Geometry: final body of the model. Coordinates: model frame, mm. Face numbers are marked on the shaded views. A direction names the side the tool comes from. Round coordinates to 2 decimals unless told otherwise and drop trailing zeros. Loops run counter-clockwise (first coordinate to the right, second up) from the corner with the lowest first, then second, coordinate; pieces in that order, holes last. Notation, with made-up numbers: (-10.5, 12.5) - (26.5, 12.5) arc R17 ccw to (26.5, 37.5) - close; hole circle Ø11 at (-14, 66). An arc over 180 degrees is marked (long way). Answer in a Markdown table with one row per item. Add a question column.
from build123d import *

# Parameters (mm, degrees)
F2_SIZE  = 1.5
F3_R     = 7
F4_DEPTH = 75.001


# Not quite as in the source:
# - a feature names something its author has since deleted; it is built from what else it names


with BuildPart() as f1:
    # F0 (on Top) → F1 (revolve)
    with BuildSketch(Plane.XY):
        with BuildLine():
            Line((-18.3783795104, 0), (31.6216204896, 0))
            Line((31.6216204896, 0), (31.6216204896, 11.5))
            Line((31.6216204896, 11.5), (53.6216204896, 11.5))
            Line((53.6216204896, 11.5), (53.6216204896, 15.2837846328))
            Line((53.6216204896, 15.2837846328), (53.6216204896, 25.2837846328))
            Line((53.6216204896, 25.2837846328), (51.6216204896, 25.2837846328))
            Line((51.6216204896, 25.2837846328), (51.6216204896, 15.2837846328))
            Line((51.6216204896, 15.2837846328), (39.6216204896, 15.2837846328))
            Line((39.6216204896, 15.2837846328), (-41.3783795104, 15.2837846328))
            Line((-41.3783795104, 15.2837846328), (-41.3783795104, 17.2837846328))
            Line((-41.3783795104, 17.2837846328), (-43.3783795104, 17.2837846328))
            Line((-43.3783795104, 17.2837846328), (-43.3783795104, 15.2837846328))
            Line((-43.3783795104, 15.2837846328), (-43.3783795104, 11.5))
            Line((-43.3783795104, 11.5), (-28.3783795104, 11.5))
            ThreePointArc((-28.3783795104, 11.5), (-21.3073116985, 8.5710678119), (-18.3783795104, 1.5))
            Line((-18.3783795104, 1.5), (-18.3783795104, 0))
        make_face()
    revolve(axis=Axis((6.6216204896, 0, 0), (-1, 0, 0)))

    # F2
    f2_edges = [f1.edges().sort_by_distance(p)[0] for p in [
        (-41.37838, -17.283785, 0),
    ]]
    chamfer(f2_edges, length=F2_SIZE)

    # F3 (on face) → F4 (cut, through all)
    with BuildSketch(Plane.YZ.offset(31.6216204896)):
        Circle(F3_R)
    extrude(amount=-F4_DEPTH, mode=Mode.SUBTRACT)


solid = f1.part
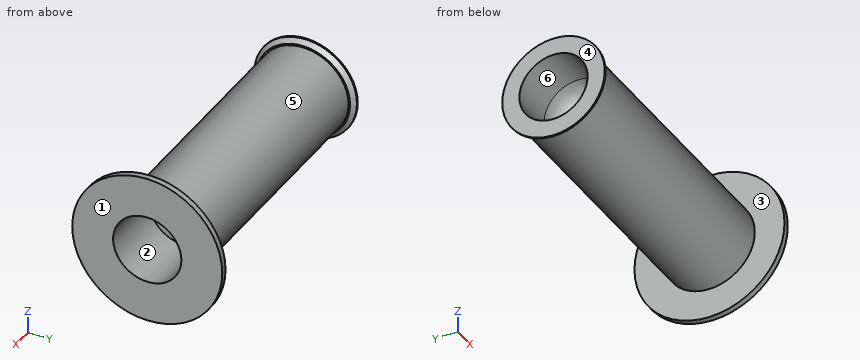
1) Pull-direction query (Z, two-part tool) for the marked faces 4, 5 and 6; classes: pulls with the +Z half, pulls with the -Z half, needs draft (parallel to the pull), parting line crosses it, or undercut.
2) Material intervals for line 1 along Z through (x, y) = (-34, 0); line 2 along Z through (x, y) = (13, 0), sorted ascending. Write a range as from..to.
3) Contact query for flat-ended pins moving along their axis: pin 1 Ø4 at (x, z) = (16.5, -16) entering from +Y; pin 2 Ø10 at (x, y) = (-21.5, 18) entering from -Z; pin 3 Ø5 at (x, y) = (33.5, -1) entering from -Z. Output: stop coordinate, or through.
4) Section B-B, the plane y = 22. Return the cut outline in (x, z), and give its area (3 significant figures).
5) Reachability of the marked faces 1, 2 and 3 from +Z, -Z, +X, -X, +Y, -Y: full face, straight path, thin tool, end or side. Return the list, or none.
6) Section A-A, the plane x = -5.5. Return the cut outline in (y, z), and give its area (3 significant figures).
Evaluation:
| question | item | result |
|---|---|---|
| 1 | face 4 | needs draft |
| 1 | face 5 | parting line crosses it |
| 1 | face 6 | undercut |
| 2 | line 1 | z = -15.28..-11.5, 11.5..15.28 |
| 2 | line 2 | z = -15.28..-7, 7..15.28 |
| 3 | pin 1 | stops at y = 6.13 |
| 3 | pin 2 | stops at z = -8.04 |
| 3 | pin 3 | stops at z = -15.28 |
| 4 | outline | (51.62, -12.46) - (53.62, -12.46) - (53.62, 12.46) - (51.62, 12.46) - close |
| 4 | area | 49.8 mm² |
| 5 | face 1 | +Z, -Z, +X, +Y, -Y |
| 5 | face 2 | +X |
| 5 | face 3 | none |
| 6 | outline | circle Ø30.57 at (0, 0); hole circle Ø14 at (0, 0) |
| 6 | area | 580 mm² |
